CAD build for the part. Positions are in the model's coordinates, mm. A direction names the side the tool comes from. Give positions to 0.01 mm unless a question says otherwise; leave off trailing zeros. Order: outer loops, then holes, each group sorted by start corner. A loop starts at its lowest first (then second) coordinate and runs counter-clockwise, first axis right, second up. Notation, with made-up numbers: M -28.5,48.25 L -2.5,48.25 A30 ccw -2.5,78.25 Z; hole C 5,76.5 d9. An arc over 180 degrees is marked long. Put each result on its own line as item: value. Start each with the question number.
1) Cut at D-D (z = 7). Write the cut outline in (x, y), and give its area (3 significant figures).
2) Two-plate mould, pull along X, no slides. Class faces 6 (the face through (-14, -38, 4)), 7 (the face through (-3.83, 16.05, 5.59)), 8 (the face through (4.83, 1.3, 3.94)): released by +X, released by -X, zero draft, split by the parting line, or undercut.
3) Cut at C-C (y = -33). Write the cut outline in (x, z).
4) Cut at A-A (z = 4). Write the cut outline in (x, y), and give its area (3 significant figures).
5) Drill centre lines: line 1 (Y direction, x = -4, z = 0.5); line 2 (Y direction, x = -3.5, z = 5.75); line 3 (Y direction, x = 3.25, z = 4). Where is each one in solid material? Low to high. Write a range as [from, to].
6) Tool access for faces 1 (the face through (-4.87, 1.14, 3.94)), 2 (the face through (0, -16, 8)), 3 (the face through (12.904, 7.648, 3.944)), 4 (the face through (-7, 16, 2)), 5 (the face through (-0.75, 13, 4)): list every direction of +Z, -Z, +X, -X, +Y, -Y with a clear straight run to the whole face (end or side of a thin tool).
7) Cut at B-B (x = -2). Write the cut outline in (y, z).
8) Pin check, flat tips, straight feed: pin 1 (6.5 mm diameter, centred on x = -7.5, y = -19, fed in from -Z); pin 2 (4 mm diameter, centred on y = 15, z = 5.5, fed in from -X); pin 3 (1 mm diameter, centred on x = 8.5, z = 6, fed in from +Y); pin 4 (3.5 mm diameter, centred on x = 7.5, y = -33, fed in from +Z) (1 decimal). Stop position of each tip, or through.
```python
from build123d import *

# Parameters (mm, degrees)
SKETCH_1_R          = 2
EXTRUDE_1_DEPTH     = 8
SKETCH_2_R          = 2
CUT_EXTRUDE_1_DEPTH = 15
FILLET_2_R          = 5


with BuildPart() as part:
    # 草图1 → 凸台-拉伸1 (new body)
    with BuildSketch(Plane.XY):
        with BuildLine():
            Line((-15, 0), (-15, -40))
            Line((-15, -40), (15, -40))
            Line((15, -40), (15, 0))
            ThreePointArc((15, 0), (12.845232579, 7.745966692), (7, 13.266499161))
            Line((7, 13.266499161), (7, 21.266499161))
            Line((7, 21.266499161), (0.75, 21.266499161))
            Line((0.75, 21.266499161), (0.75, 4.943429983))
            ThreePointArc((0.75, 4.943429983), (4.848902965, 1.219893452), (3, -4))
            Line((3, -4), (-3, -4))
            ThreePointArc((-3, -4), (-4.848902965, 1.219893452), (-0.75, 4.943429983))
            Line((-0.75, 4.943429983), (-0.75, 21.266499161))
            Line((-0.75, 21.266499161), (-7, 21.266499161))
            Line((-7, 21.266499161), (-7, 13.266499161))
            ThreePointArc((-7, 13.266499161), (-12.845232579, 7.745966692), (-15, 0))
        make_face()
        with Locations((-7.5, -19)):
            Circle(SKETCH_1_R, mode=Mode.SUBTRACT)
        with Locations((-7.5, -33)):
            Circle(SKETCH_1_R, mode=Mode.SUBTRACT)
        with Locations(Location((7.5, -33, 0), (0, 0, 180))):
            Circle(SKETCH_1_R, mode=Mode.SUBTRACT)
        with Locations(Location((7.5, -19, 0), (0, 0, 180))):
            Circle(SKETCH_1_R, mode=Mode.SUBTRACT)
    extrude(amount=EXTRUDE_1_DEPTH)

    # 草图2 → 切除-拉伸1 (cut)
    with BuildSketch(Plane(origin=(7, 0, 0), x_dir=(0, 0, -1), z_dir=(1, 0, 0))):
        with Locations((-4, 17.266499161)):
            Circle(SKETCH_2_R)
    extrude(amount=-CUT_EXTRUDE_1_DEPTH, mode=Mode.SUBTRACT)

    # 圆角2
    fillet_2_edges = [part.edges().sort_by_distance(p)[0] for p in [
        (15, -40, 4),
        (-15, -40, 4),
    ]]
    fillet(fillet_2_edges, radius=FILLET_2_R)


solid = part.part
```
Solution:
1. outline: M -15,-35 A5 ccw -10,-40 L 10,-40 A5 ccw 15,-35 L 15,0 A15 ccw 7,13.27 L 7,21.27 L 0.75,21.27 L 0.75,4.94 A5 cw 3,-4 L -3,-4 A5 cw -0.75,4.94 L -0.75,21.27 L -7,21.27 L -7,13.27 A15 ccw -15,0 Z; hole C -7.5,-33 d4; hole C -7.5,-19 d4; hole C 7.5,-33 d4; hole C 7.5,-19 d4
1. area: 1,490 mm²
2. face 6: released by -X
2. face 7: zero draft
2. face 8: undercut
3. outline: M -15,0 L -9.5,0 L -9.5,8 L -15,8 Z; M -5.5,0 L 5.5,0 L 5.5,8 L -5.5,8 Z; M 9.5,0 L 15,0 L 15,8 L 9.5,8 Z
4. outline: M -15,-35 A5 ccw -10,-40 L 10,-40 A5 ccw 15,-35 L 15,0 A15 ccw 7,13.27 L 7,15.27 L 0.75,15.27 L 0.75,4.94 A5 cw 3,-4 L -3,-4 A5 cw -0.75,4.94 L -0.75,15.27 L -7,15.27 L -7,13.27 A15 ccw -15,0 Z; M -7,19.27 L -0.75,19.27 L -0.75,21.27 L -7,21.27 Z; M 0.75,19.27 L 7,19.27 L 7,21.27 L 0.75,21.27 Z; hole C -7.5,-33 d4; hole C -7.5,-19 d4; hole C 7.5,-33 d4; hole C 7.5,-19 d4
4. area: 1,440 mm²
5. line 1: [-40, -3], [3, 21.27]
5. line 2: [-40, -3.57], [3.57, 16.3], [18.23, 21.27]
5. line 3: [-40, -3.8], [3.8, 15.27], [19.27, 21.27]
6. face 1: +Z, -Z
6. face 2: +Z, +X, -X, +Y, -Y
6. face 3: +Z, -Z, +X, +Y
6. face 4: +Z, -Z, -X, +Y
6. face 5: +Z, -Z, +Y
7. outline: M -40,0 L -4,0 L -4,8 L -40,8 Z; M 4.58,0 L 21.27,0 L 21.27,8 L 4.58,8 Z; hole C 17.27,4 d4
8. pin 1: z = 0
8. pin 2: x = -7.48
8. pin 3: y = 12.69
8. pin 4: through
